from build123d import *

# Parameters (mm, degrees)
ESQUISSE1_W                = 28.3
ESQUISSE1_H                = 28.3
ESQUISSE1_W_2              = 20.3
ESQUISSE1_H_2              = 20.3
ESQUISSE1_W_3              = 4
ESQUISSE1_H_3              = 2
BOSS_EXTRU_1_DEPTH         = 20
BOSS_EXTRU_7_DEPTH         = 20
ESQUISSE2_W                = 8.5
ESQUISSE2_H                = 20
ESQUISSE2_R                = 1.7
BOSS_EXTRU_2_DEPTH         = 2
ESQUISSE2_3_W              = 8.5
ESQUISSE2_3_H              = 20
BOSS_EXTRU_3_DEPTH         = 3
ESQUISSE3_W                = 8.5
ESQUISSE3_H                = 20
ESQUISSE3_R                = 1.7
BOSS_EXTRU_4_DEPTH         = 2
ESQUISSE5_W                = 8.5
ESQUISSE5_H                = 20
ESQUISSE5_R                = 3
BOSS_EXTRU_5_DEPTH         = 2
BOSS_EXTRU_6_DEPTH         = 20
BOSS_EXTRU_6_DEPTH_BACK    = 20
ESQUISSE6_W                = 28.3
ESQUISSE6_H                = 28.3
ESQUISSE6_W_2              = 15.3
ESQUISSE6_H_2              = 15.3
ENL_V_MAT_EXTRU_1_REACH    = 68.678
ESQUISSE7_W                = 6.5
ESQUISSE7_H                = 2
ENL_V_MAT_EXTRU_2_REACH    = 65.341
ESQUISSE8_W                = 14.15
ESQUISSE8_H                = 2
ESQUISSE9_W                = 8.5
ESQUISSE9_H                = 40
BOSS_EXTRU_8_DEPTH         = 5
ESQUISSE9_4_R              = 1.7
BOSS_EXTRU_9_DEPTH         = 2
BOSS_EXTRU_10_START        = -2
ESQUISSE10_W               = 8.5
ESQUISSE10_H               = 40
ESQUISSE10_R               = 1.7
BOSS_EXTRU_10_DEPTH        = 2
ESQUISSE11_W               = 8.5
ESQUISSE11_H               = 40
ESQUISSE11_R               = 3
BOSS_EXTRU_11_DEPTH        = 2
NERVURE4_REACH             = 68.678
ESQUISSE14_WALL_W          = 147.131281186
ESQUISSE14_WALL_H          = 5
NERVURE10_REACH            = 68.678
ESQUISSE16_WALL_W          = 147.844247416
ESQUISSE16_WALL_H          = 5
R_P_TITION_LIN_AIRE1_COUNT = 3
R_P_TITION_LIN_AIRE1_PITCH = 17.5
NERVURE11_REACH            = 76.685
ESQUISSE17_WALL_W          = 163.85974229
ESQUISSE17_WALL_H          = 5
NERVURE17_REACH            = 58.973
ESQUISSE19_WALL_W          = 127.721749296
ESQUISSE19_WALL_H          = 5
R_P_TITION_LIN_AIRE2_COUNT = 2
R_P_TITION_LIN_AIRE2_PITCH = 15
R_P_TITION_LIN_AIRE3_COUNT = 2
R_P_TITION_LIN_AIRE3_PITCH = 15
ENL_V_MAT_EXTRU_3_REACH    = 52.13
ESQUISSE20_W               = 77.833771897
ESQUISSE20_H               = 63.25162408
ESQUISSE21_W               = 120
ESQUISSE21_H               = 100
BOSS_EXTRU_12_DEPTH        = 5
CHANFREIN1_SIZE            = 10


with BuildPart() as part:
    # Esquisse1 → Boss.-Extru.1 (new body)
    # profile 1 of 2: a face of its own
    with BuildSketch(Plane.XY):
        Rectangle(ESQUISSE1_W, ESQUISSE1_H)
        Rectangle(ESQUISSE1_W_2, ESQUISSE1_H_2, mode=Mode.SUBTRACT)
    # profile 2 of 2: a face of its own
    with BuildSketch(Plane.XY):
        with Locations((12.15, -1)):
            Rectangle(ESQUISSE1_W_3, ESQUISSE1_H_3)
    extrude(amount=BOSS_EXTRU_1_DEPTH)

    # Esquisse1<3> → Boss.-Extru.7 (add)
    with BuildSketch(Plane.XY):
        Polygon((14.15, 14.15), (-14.15, 14.15), (-14.15, -14.15), (14.15, -14.15), (14.15, -2), (10.15, -2), (10.15, -10.15), (-10.15, -10.15), (-10.15, 10.15), (10.15, 10.15), (10.15, 0), (14.15, 0), align=None)
    extrude(amount=-BOSS_EXTRU_7_DEPTH)

    # Esquisse2 → Boss.-Extru.2 (add)
    with BuildSketch(Plane(origin=(0, 2, 0), x_dir=(-1, 0, 0), z_dir=(0, -1, 0))):
        with Locations((-18.4, 10)):
            Rectangle(ESQUISSE2_W, ESQUISSE2_H)
        with Locations(Location((-18.4, 10, 0), (0, 0, 180))):
            Circle(ESQUISSE2_R, mode=Mode.SUBTRACT)
    extrude(amount=BOSS_EXTRU_2_DEPTH)

    # Esquisse2<3> → Boss.-Extru.3 (add)
    with BuildSketch(Plane(origin=(0, 2, 0), x_dir=(-1, 0, 0), z_dir=(0, -1, 0))):
        with Locations((-18.4, 10)):
            Rectangle(ESQUISSE2_3_W, ESQUISSE2_3_H)
        Polygon((-15.65, 11.58771324), (-15.65, 8.41228676), (-18.4, 6.824573519), (-21.15, 8.41228676), (-21.15, 11.58771324), (-18.4, 13.175426481), align=None, mode=Mode.SUBTRACT)
    extrude(amount=-BOSS_EXTRU_3_DEPTH)

    # Esquisse3 → Boss.-Extru.4 (add)
    with BuildSketch(Plane(origin=(0, -2, 0), x_dir=(1, 0, 0), z_dir=(0, 1, 0))):
        with Locations((18.4, 10)):
            Rectangle(ESQUISSE3_W, ESQUISSE3_H)
        with Locations((18.4, 10)):
            Circle(ESQUISSE3_R, mode=Mode.SUBTRACT)
    extrude(amount=-BOSS_EXTRU_4_DEPTH)

    # Esquisse5 → Boss.-Extru.5 (add)
    with BuildSketch(Plane.XZ.offset(4)):
        with Locations((18.4, -10)):
            Rectangle(ESQUISSE5_W, ESQUISSE5_H)
        with Locations((18.4, -10)):
            Circle(ESQUISSE5_R, mode=Mode.SUBTRACT)
    extrude(amount=BOSS_EXTRU_5_DEPTH)

    # Esquisse6 → Boss.-Extru.6 (add, two sides: drawn at the far end of the back side and taken through both)
    with BuildSketch(Plane(origin=(0, 0, 0), x_dir=(-1, 0, 0), z_dir=(0, -1, 0)).offset(-BOSS_EXTRU_6_DEPTH_BACK)):
        with Locations((0, -34.15)):
            Rectangle(ESQUISSE6_W, ESQUISSE6_H)
        with Locations((0, -34.15)):
            Rectangle(ESQUISSE6_W_2, ESQUISSE6_H_2, mode=Mode.SUBTRACT)
    extrude(amount=BOSS_EXTRU_6_DEPTH + BOSS_EXTRU_6_DEPTH_BACK)

    # Esquisse7 → Enlèv. mat.-Extru.1 (cut, up to next)
    with BuildSketch(Plane.XZ.offset(20), mode=Mode.PRIVATE) as enl_v_mat_extru_1_sk1:
        with Locations((10.9, 35.15)):
            Rectangle(ESQUISSE7_W, ESQUISSE7_H)
    enl_v_mat_extru_1_tool1 = extrude(enl_v_mat_extru_1_sk1.sketch, amount=-ENL_V_MAT_EXTRU_1_REACH, mode=Mode.PRIVATE) & part.part
    add(enl_v_mat_extru_1_tool1.solids().sort_by_distance((10.9, -20, 35.15))[0], mode=Mode.SUBTRACT)

    # Esquisse8 → Enlèv. mat.-Extru.2 (cut, up to next)
    with BuildSketch(Plane.XZ.offset(14.15), mode=Mode.PRIVATE) as enl_v_mat_extru_2_sk1:
        with Locations((7.075, 1)):
            Rectangle(ESQUISSE8_W, ESQUISSE8_H)
    enl_v_mat_extru_2_tool1 = extrude(enl_v_mat_extru_2_sk1.sketch, amount=-ENL_V_MAT_EXTRU_2_REACH, mode=Mode.PRIVATE) & part.part
    add(enl_v_mat_extru_2_tool1.solids().sort_by_distance((7.075, -14.15, 1))[0], mode=Mode.SUBTRACT)

    # Esquisse9 → Boss.-Extru.8 (add)
    with BuildSketch(Plane.XY.offset(34.15)):
        with Locations((18.4, 0)):
            Rectangle(ESQUISSE9_W, ESQUISSE9_H)
        Polygon((18.4, 6.824573519), (21.15, 8.41228676), (21.15, 11.58771324), (18.4, 13.175426481), (15.65, 11.58771324), (15.65, 8.41228676), align=None, mode=Mode.SUBTRACT)
        Polygon((18.4, -6.824573519), (21.15, -8.41228676), (21.15, -11.58771324), (18.4, -13.175426481), (15.65, -11.58771324), (15.65, -8.41228676), align=None, mode=Mode.SUBTRACT)
    extrude(amount=-BOSS_EXTRU_8_DEPTH)

    # Esquisse9<4> → Boss.-Extru.9 (add)
    # profile 1 of 2: a face of its own
    with BuildSketch(Plane.XY.offset(34.15)):
        Polygon((15.65, 8.41228676), (18.4, 6.824573519), (21.15, 8.41228676), (21.15, 11.58771324), (18.4, 13.175426481), (15.65, 11.58771324), align=None)
        with Locations((18.4, 10)):
            Circle(ESQUISSE9_4_R, mode=Mode.SUBTRACT)
    # profile 2 of 2: a face of its own
    with BuildSketch(Plane.XY.offset(34.15)):
        Polygon((21.15, -8.41228676), (21.15, -11.58771324), (18.4, -13.175426481), (15.65, -11.58771324), (15.65, -8.41228676), (18.4, -6.824573519), align=None)
        with Locations((18.4, -10)):
            Circle(ESQUISSE9_4_R, mode=Mode.SUBTRACT)
    extrude(amount=-BOSS_EXTRU_9_DEPTH)

    # Esquisse10 → Boss.-Extru.10 (add)
    with BuildSketch(Plane(origin=(0, 0, 36.15), x_dir=(-1, 0, 0), z_dir=(0, 0, -1)).offset(BOSS_EXTRU_10_START)):
        with Locations((-18.4, 0)):
            Rectangle(ESQUISSE10_W, ESQUISSE10_H)
        with Locations(Location((-18.4, -10, 0), (0, 0, 180))):
            Circle(ESQUISSE10_R, mode=Mode.SUBTRACT)
        with Locations(Location((-18.4, 10, 0), (0, 0, 180))):
            Circle(ESQUISSE10_R, mode=Mode.SUBTRACT)
    extrude(amount=BOSS_EXTRU_10_DEPTH)

    # Esquisse11 → Boss.-Extru.11 (add)
    with BuildSketch(Plane.XY.offset(38.15)):
        with Locations((18.4, 0)):
            Rectangle(ESQUISSE11_W, ESQUISSE11_H)
        with Locations((18.4, 10)):
            Circle(ESQUISSE11_R, mode=Mode.SUBTRACT)
        with Locations((18.4, -10)):
            Circle(ESQUISSE11_R, mode=Mode.SUBTRACT)
    extrude(amount=BOSS_EXTRU_11_DEPTH)

    # Esquisse14 wall → Nervure4 (add, up to next)
    with BuildSketch(Plane(origin=(18.4, -20, 44.225), x_dir=(0.721811427095, 0, -0.692089780097), z_dir=(0.692089780097, 0, 0.721811427095)), mode=Mode.PRIVATE) as nervure4_sk1:
        with Locations((0, 2.5)):
            Rectangle(ESQUISSE14_WALL_W, ESQUISSE14_WALL_H)
    nervure4_tool1 = extrude(nervure4_sk1.sketch, amount=-NERVURE4_REACH, mode=Mode.PRIVATE) - part.part
    nervure4 = nervure4_tool1.solids().sort_by_distance((18.4, -20, 44.225))[0]
    add(nervure4)

    # Esquisse16 wall → Nervure10 (add, up to next)
    with BuildSketch(Plane(origin=(18.4, -20, 24.575), x_dir=(-0.680604645507, 0, -0.732650883105), z_dir=(0.732650883105, 0, -0.680604645507)), mode=Mode.PRIVATE) as nervure10_sk1:
        with Locations((0, 2.5)):
            Rectangle(ESQUISSE16_WALL_W, ESQUISSE16_WALL_H)
    nervure10_tool1 = extrude(nervure10_sk1.sketch, amount=-NERVURE10_REACH, mode=Mode.PRIVATE) - part.part
    nervure10 = nervure10_tool1.solids().sort_by_distance((18.4, -20, 24.575))[0]
    add(nervure10)

    # Répétition linéaire1: Nervure4, Nervure10 ×3
    with Locations(*[(0, i * R_P_TITION_LIN_AIRE1_PITCH, 0) for i in range(1, R_P_TITION_LIN_AIRE1_COUNT)]):
        add(nervure4)
        add(nervure10)

    # Esquisse17 wall → Nervure11 (add, up to next)
    with BuildSketch(Plane(origin=(18.4, 9.575, -20), x_dir=(-0.680604645507, 0.732650883105, 0), z_dir=(0.732650883105, 0.680604645507, 0)), mode=Mode.PRIVATE) as nervure11_sk1:
        with Locations((0, 2.5)):
            Rectangle(ESQUISSE17_WALL_W, ESQUISSE17_WALL_H)
    nervure11_tool1 = extrude(nervure11_sk1.sketch, amount=-NERVURE11_REACH, mode=Mode.PRIVATE) - part.part
    nervure11 = nervure11_tool1.solids().sort_by_distance((18.4, 9.575, -20))[0]
    add(nervure11)

    # Esquisse19 wall → Nervure17 (add, up to next)
    with BuildSketch(Plane(origin=(18.4, -10.075, 0), x_dir=(-0.721811427095, -0.692089780097, 0), z_dir=(0.692089780097, -0.721811427095, 0)), mode=Mode.PRIVATE) as nervure17_sk1:
        with Locations((0, 2.5)):
            Rectangle(ESQUISSE19_WALL_W, ESQUISSE19_WALL_H)
    nervure17_tool1 = extrude(nervure17_sk1.sketch, amount=-NERVURE17_REACH, mode=Mode.PRIVATE) - part.part
    nervure17 = nervure17_tool1.solids().sort_by_distance((18.4, -10.075, 0))[0]
    add(nervure17)

    # Répétition linéaire2: Nervure17 ×2
    with Locations(*[(0, 0, -i * R_P_TITION_LIN_AIRE2_PITCH) for i in range(1, R_P_TITION_LIN_AIRE2_COUNT)]):
        add(nervure17)

    # Répétition linéaire3: Nervure11 ×2
    with Locations(*[(0, 0, i * R_P_TITION_LIN_AIRE3_PITCH) for i in range(1, R_P_TITION_LIN_AIRE3_COUNT)]):
        add(nervure11)

    # Esquisse20 → Enlèv. mat.-Extru.3 (cut, up to next)
    with BuildSketch(Plane(origin=(0, 0, 20), x_dir=(-1, 0, 0), z_dir=(0, 0, -1)), mode=Mode.PRIVATE) as enl_v_mat_extru_3_sk1:
        with Locations((6.593135557, -7.228757038)):
            Rectangle(ESQUISSE20_W, ESQUISSE20_H)
    enl_v_mat_extru_3_tool1 = extrude(enl_v_mat_extru_3_sk1.sketch, amount=-ENL_V_MAT_EXTRU_3_REACH, mode=Mode.PRIVATE) & part.part
    add(enl_v_mat_extru_3_tool1.solids().sort_by_distance((-6.593136, -7.228757, 20))[0], mode=Mode.SUBTRACT)

    # Esquisse21 → Boss.-Extru.12 (add)
    with BuildSketch(Plane.XY.offset(20)):
        with Locations((9.5, 35)):
            Rectangle(ESQUISSE21_W, ESQUISSE21_H)
    extrude(amount=BOSS_EXTRU_12_DEPTH)

    # Chanfrein1
    chanfrein1_edges = [part.edges().sort_by_distance(p)[0] for p in [
        (0, 14.15, 20),
        (14.15, 0, 20),
        (-14.15, 0, 20),
    ]]
    chamfer(chanfrein1_edges, length=CHANFREIN1_SIZE)


solid = part.part
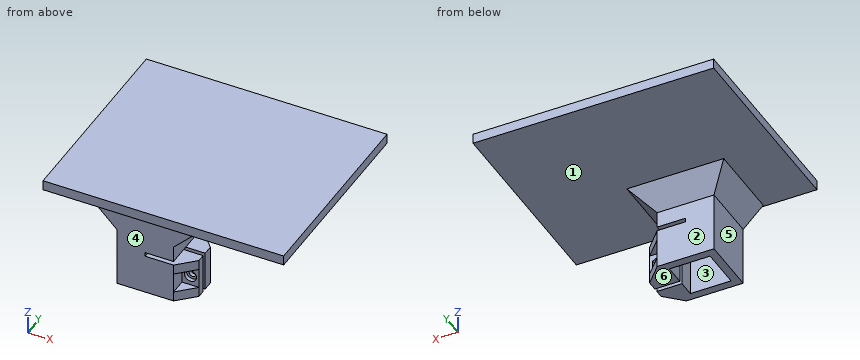
Here's how the part is built. I have some questions about the finished solid (model axes, mm). Face numbers are marked on the shaded views. A direction names the side the tool comes from. Round coordinates to 2 decimals unless told otherwise and drop trailing zeros. Order: outer loops, then holes, each group sorted by start corner. A loop starts at its lowest first (then second) coordinate and runs counter-clockwise, first axis right, second up. Notation, with made-up numbers: M -18.5,2.5 L 17.5,2.5 A32 ccw 17.5,36.5 Z; hole C -12,-30 d1. An arc over 180 degrees is marked long. Return JSON: item names as keys, results as strings. Group by question number.
1. If we section it at B-B on z = 5: List the corners of the cut face in (x, y) for me, then the cut area to 3 significant figures.
2. If we mould it in two halves opening along Y, with no side actions, what happens to the marked faces 1, 2 and 3? For each: pulls with the +Y half, pulls with the -Y half, needs draft (parallel to the pull), parting line crosses it, or undercut.
3. If we section it at C-C on x = 3.5: List the corners of the cut face in (y, z) for me, then the cut area to 3 significant figures.
4. Please list where these lines run through material, in increasing order: probe 1 along X at (y, z) = (-3.35, -10); probe 2 along Y at (x, z) = (7, 2.5); probe 3 along Z at (x, y) = (18.4, -3.05).
5. On a 3-axis mill with a long thin cutter (end or side, diameter ignored), from which of +Z, -Z, +X, -X, +Y, -Y can I reach the whole of each face in a straight line? I mean the marked faces 4, 5 and 6. Say none if no direction works.
6. If we section it at A-A on z = -10: State how many separate pieces and enclosed holes the cut face has, then the cut area to 3 significant figures.
7. If we section it at D-D on x = 29: List the corners of the cut face in (y, z) for me.
8. I'm going to push flat-ended pins straight in: pin 1 Ø2 at (y, z) = (-3.5, -13) entering from +X; pin 2 Ø4.5 at (x, z) = (19.5, -11) entering from +Y; pin 3 Ø16 at (x, y) = (-1, -2) entering from -Z. Where does each tip first touch, or does it pass through?
Reply:
{
 "1": {"outline": "M -14.15,-14.15 L 14.15,-14.15 L 14.15,14.15 L -14.15,14.15 Z; hole M -10.15,-10.15 L 10.15,-10.15 L 10.15,10.15 L -10.15,10.15 Z", "area": "389 mm^2"},
 "2": {"face 1": "needs draft", "face 2": "pulls with the +Y half", "face 3": "undercut"},
 "3": {"outline": "M -15,20 L -14.15,20 L -14.15,2 L -10.15,2 L -10.15,20 L 10.15,20 L 10.15,2 L 14.15,2 L 14.15,10 L 24.15,20 L 85,20 L 85,25 L -15,25 Z; M -14.15,-20 L -10.15,-20 L -10.15,0 L -14.15,0 Z; M 10.15,-20 L 14.15,-20 L 14.15,0 L 10.15,0 Z", "area": "854 mm^2"},
 "4": {"probe 1": "-14.15 to -10.15, 10.15 to 16.7, 20.1 to 22.65", "probe 2": "-14.15 to -10.15, 10.15 to 14.15", "probe 3": "-20 to -11.7, -8.3 to 0, 14.25 to 25"},
 "5": {"face 4": "-Z, +X, -X, -Y", "face 5": "-Z, -X, +Y, -Y", "face 6": "-Z, +X, -X, +Y, -Y"},
 "6": {"separate pieces": "3", "enclosed holes": "0", "area": "415 mm^2"},
 "7": {"outline": "M -15,20 L 85,20 L 85,25 L -15,25 Z"},
 "8": {"pin 1": "x = 22.65", "pin 2": "y = 5", "pin 3": "z = 20"}
}
